Design review of the part built by this model. Coordinates are the model's own, in mm. Coordinates: 2 decimals unless noted, no trailing zeros. Write each loop counter-clockwise with the first axis right and the second up, starting at its lowest first coordinate (ties: lowest second). Pieces come first, ordered by that corner, then holes. Notation, with made-up numbers: (24, 24) -> (75, 24) arc R14 cw to (75, 38) -> close; hole circle Ø1 at (58, 20.25). An arc over 180 degrees is marked (long way). Return JSON: item names as keys, results as strings. Group by question number.
from build123d import *

# Parameters (mm, degrees)
SKETCH_1_R      = 2
SKETCH_1_R_2    = 50
EXTRUDE_1_DEPTH = 4
FILLET_1_R      = 10


with BuildPart() as part:
    # 草图1 → 凸台-拉伸1 (new body)
    with BuildSketch(Plane(origin=(0, 0, 0), x_dir=(1, 0, 0), z_dir=(0, 1, 0))):
        Polygon((25, 85), (-25, 85), (-85, 25), (-85, -25), (-25, -85), (25, -85), (85, -25), (85, 25), align=None)
        with Locations(Location((-15, -75, 0), (0, 0, 270))):
            Circle(SKETCH_1_R, mode=Mode.SUBTRACT)
        with Locations(Location((-15, -60, 0), (0, 0, 270))):
            Circle(SKETCH_1_R, mode=Mode.SUBTRACT)
        with Locations(Location((-75, -15, 0), (0, 0, 270))):
            Circle(SKETCH_1_R, mode=Mode.SUBTRACT)
        with Locations(Location((-60, -15, 0), (0, 0, 270))):
            Circle(SKETCH_1_R, mode=Mode.SUBTRACT)
        with Locations(Location((15, -75, 0), (0, 0, 270))):
            Circle(SKETCH_1_R, mode=Mode.SUBTRACT)
        with Locations(Location((15, -60, 0), (0, 0, 270))):
            Circle(SKETCH_1_R, mode=Mode.SUBTRACT)
        with Locations(Location((0, 0, 0), (0, 0, 270))):
            Circle(SKETCH_1_R_2, mode=Mode.SUBTRACT)
        with Locations(Location((60, -15, 0), (0, 0, 270))):
            Circle(SKETCH_1_R, mode=Mode.SUBTRACT)
        with Locations(Location((75, -15, 0), (0, 0, 270))):
            Circle(SKETCH_1_R, mode=Mode.SUBTRACT)
        with Locations(Location((-75, 15, 0), (0, 0, 270))):
            Circle(SKETCH_1_R, mode=Mode.SUBTRACT)
        with Locations(Location((-60, 15, 0), (0, 0, 270))):
            Circle(SKETCH_1_R, mode=Mode.SUBTRACT)
        with Locations(Location((-15, 60, 0), (0, 0, 270))):
            Circle(SKETCH_1_R, mode=Mode.SUBTRACT)
        with Locations(Location((-15, 75, 0), (0, 0, 270))):
            Circle(SKETCH_1_R, mode=Mode.SUBTRACT)
        with Locations(Location((60, 15, 0), (0, 0, 270))):
            Circle(SKETCH_1_R, mode=Mode.SUBTRACT)
        with Locations(Location((75, 15, 0), (0, 0, 270))):
            Circle(SKETCH_1_R, mode=Mode.SUBTRACT)
        with Locations(Location((15, 60, 0), (0, 0, 270))):
            Circle(SKETCH_1_R, mode=Mode.SUBTRACT)
        with Locations(Location((15, 75, 0), (0, 0, 270))):
            Circle(SKETCH_1_R, mode=Mode.SUBTRACT)
    extrude(amount=EXTRUDE_1_DEPTH)

    # 圆角1
    fillet_1_edges = [part.edges().sort_by_distance(p)[0] for p in [
        (-25, 2, 85),
        (-85, 2, 25),
        (-85, 2, -25),
        (-25, 2, -85),
        (25, 2, -85),
        (85, 2, -25),
        (85, 2, 25),
        (25, 2, 85),
    ]]
    fillet(fillet_1_edges, radius=FILLET_1_R)


solid = part.part
Q1. Wall thickness on L1, parallel to X at y = 3, z = 60; L2, parallel to X at y = 1.3, z = 15; L3, parallel to X at y = 2.95, z = 59: over which ranges is each line inside the solid? List them lowest first.
Q2. We need section A-A on x = 0. Write out the cut boundary in (y, z).
Q3. We need section B-B on z = 60. Write out the cut boundary in (x, y).
Q4. We need section D-D on x = -60. Write out the cut boundary in (y, z), plus the area to 3 significant figures.
Q5. We need section C-C on y = 0.9. State how many separate pieces and enclosed holes the cut face has, plus the area to 3 significant figures.
Q6. The part is to be moulded in two halves that separate along X. For faces 1 (the flat face through (55, 2, 55)), 2 (the flat face through (0, 2, 85)), 3 (the cylindrical face through (17, 2, 60)), say which applies: +X half, -X half, draft (parallel to the pull), parting line (faces both ways), or undercut.
Q7. For P1, Ø2, axis at y = 2, z = 56.5, coming from the -X side, flat-tipped, find the tip position at first contact; note if it passes through.
Findings below:
{
 "1": {"L1": "x = -50 to -17, -13 to 13, 17 to 50", "L2": "x = -85 to -77, -73 to -62, -58 to -47.7, 47.7 to 58, 62 to 73, 77 to 85", "L3": "x = -51 to -16.73, -13.27 to 13.27, 16.73 to 51"},
 "2": {"outline": "(0, -85) -> (4, -85) -> (4, -50) -> (0, -50) -> close; (0, 50) -> (4, 50) -> (4, 85) -> (0, 85) -> close"},
 "3": {"outline": "(-50, 0) -> (-17, 0) -> (-17, 4) -> (-50, 4) -> close; (-13, 0) -> (13, 0) -> (13, 4) -> (-13, 4) -> close; (17, 0) -> (50, 0) -> (50, 4) -> (17, 4) -> close"},
 "4": {"outline": "(0, -50) -> (4, -50) -> (4, -17) -> (0, -17) -> close; (0, -13) -> (4, -13) -> (4, 13) -> (0, 13) -> close; (0, 17) -> (4, 17) -> (4, 50) -> (0, 50) -> close", "area": "368 mm^2"},
 "5": {"separate pieces": "1", "enclosed holes": "17", "area": "13,600 mm^2"},
 "6": {"face 1": "+X half", "face 2": "draft", "face 3": "undercut"},
 "7": {"P1": "stops at x = -54.5"}
}
